from build123d import *

# Parameters (mm, degrees)
SKETCH1_R           = 7.112
BOSS_EXTRUDE1_DEPTH = 5.1435
SKETCH2_2_R         = 4.6228
BOSS_EXTRUDE2_DEPTH = 7.366
SKETCH4_R           = 7.01675
BOSS_EXTRUDE3_DEPTH = 1.2446
SKETCH6_R           = 2.39395
CUT_EXTRUDE1_DEPTH  = 18.576657848


with BuildPart() as part:
    # Sketch1 → Boss-Extrude1 (new body)
    with BuildSketch(Plane.XY):
        Circle(SKETCH1_R)
    extrude(amount=-BOSS_EXTRUDE1_DEPTH)

    # Loft1: read off the stored shape, not the designer's step
    # Loft1: loft between two sections, ruled curve by curve
    loft1_from = [
        Edge.make_bspline([(6.805435292, 2.065573645, 0), (2.674288001, 15.67644423, 0), (-10.936582583, 11.545296939, 0), (-6.805435292, -2.065573645, 0), (-2.674288001, -15.67644423, 0), (10.936582583, -11.545296939, 0), (6.805435292, 2.065573645, 0)], [0, 0, 0, 0, 0.5, 0.5, 0.5, 1, 1, 1, 1], 3, [1, 0.333333333, 0.333333333, 1, 0.333333333, 0.333333333, 1]),
    ]
    loft1_to = [
        Edge.make_bspline([(4.035501617, 2.254995907, 0.6604), (-0.474490196, 10.325999141, 0.6604), (-8.54549343, 5.816007327, 0.6604), (-4.035501617, -2.254995907, 0.6604), (0.474490196, -10.325999141, 0.6604), (8.54549343, -5.816007327, 0.6604), (4.035501617, 2.254995907, 0.6604)], [0, 0, 0, 0, 0.5, 0.5, 0.5, 1, 1, 1, 1], 3, [1, 0.333333333, 0.333333333, 1, 0.333333333, 0.333333333, 1]),
    ]
    loft1 = Solid(Shell([*[Face.make_surface_from_curves(loft1_from[k], loft1_to[k]) for k in range(1)], Face(Wire(loft1_from)), Face(Wire(loft1_to))]))
    add(loft1)

    # Sketch2<2> → Boss-Extrude2 (add)
    with BuildSketch(Plane.XY.offset(0.6604)):
        with Locations(Location((0, 0, 0), (0, 0, 29.196))):
            Circle(SKETCH2_2_R)
    extrude(amount=BOSS_EXTRUDE2_DEPTH)

    # Sketch4 → Boss-Extrude3 (add)
    with BuildSketch(Plane.XY.offset(8.0264)):
        Circle(SKETCH4_R)
    extrude(amount=BOSS_EXTRUDE3_DEPTH)

    # Sketch6 → Cut-Extrude1 (cut, through all)
    with BuildSketch(Plane(origin=(0, 0, -5.1435), x_dir=(-1, 0, 0), z_dir=(0, 0, -1))):
        Circle(SKETCH6_R)
    extrude(amount=-CUT_EXTRUDE1_DEPTH, mode=Mode.SUBTRACT)


solid = part.part
Input: part model. Units: mm. Frame: model coordinates. A direction names the side the tool comes from. Coordinates: 2 decimals unless noted, no trailing zeros. Loops run counter-clockwise (first coordinate to the right, second up) from the corner with the lowest first, then second, coordinate; pieces in that order, holes last.
Q1. Set-up query: faces 4 (the face through (3.172, 3.363, 4.292)), 5 (the face through (-1.542, -6.943, -2.536)). Return all of +Z, -Z, +X, -X, +Y, -Y with unobstructed straight access to the full face (end or side cutting, diameter ignored); none if empty.
Q2. Cut plane A-A (z = -3.25). Output: boundary loops of the cut face in (x, y), then the cut area to 3 significant figures.
Q3. Draft query along Z for faces 1 (the face through (1, -5, 8.026)), 2 (the face through (-5.172, 4.742, 8.64)), 3 (the face through (0, -3, 9.271)). Return one class per face: +Z half, -Z half, draft (parallel to the pull), parting line (faces both ways), or undercut.
Q4. Material intervals for line 1 (Y direction, x = 0, z = -1); line 2 (Y direction, x = 0, z = 6.5); line 3 (Z direction, x = -4.5, y = 5.25), sorted ascending.
Q5. Contact query for flat-ended pins moving along their axis: pin 1 (3 mm diameter, centred on x = -1.5, y = -0.5, fed in from -Z); pin 2 (6 mm diameter, centred on y = 3.5, z = 7, fed in from +X); pin 3 (4 mm diameter, centred on x = -4, z = 8, fed in from -Y). Output: stop coordinate, or through.
Q6. Cut plane B-B (z = 3.5). Output: boundary loops of the cut face in (x, y) (1 decimal), then the cut area to 3 significant figures.
Working result:
1. face 4: none
1. face 5: +Z, -Z
2. outline: circle Ø14.22 at (0, 0); hole circle Ø4.79 at (0, 0)
2. area: 141 mm2
3. face 1: undercut
3. face 2: draft
3. face 3: +Z half
4. line 1: y = -7.11 to -2.39, 2.39 to 7.11
4. line 2: y = -4.62 to -2.39, 2.39 to 4.62
4. line 3: z = -5.14 to 0.05, 8.03 to 9.27
5. pin 1: stops at z = -5.14
5. pin 2: stops at x = 6.98
5. pin 3: stops at y = -6.73
6. outline: circle Ø9.2 at (0, 0); hole circle Ø4.8 at (0, 0)
6. area: 49.1 mm2
